CAD build for the part. Positions are in the model's coordinates, mm. A direction names the side the tool comes from. Give positions to 0.01 mm unless a question says otherwise; leave off trailing zeros. Loops run counter-clockwise (first coordinate to the right, second up) from the corner with the lowest first, then second, coordinate; pieces in that order, holes last.
```python
from build123d import *

# Parameters (mm, degrees)
SKETCH1_R           = 44.45
BOSS_EXTRUDE1_DEPTH = 6.35
BOSS_EXTRUDE4_DEPTH = 34.036
SKETCH3_R           = 2.6416
CUT_EXTRUDE1_DEPTH  = 75.717026145


with BuildPart() as part:
    # Sketch1 → Boss-Extrude1 (new body)
    with BuildSketch(Plane.XY):
        Circle(SKETCH1_R)
    extrude(amount=BOSS_EXTRUDE1_DEPTH)

    # Sketch2 → Boss-Extrude4 (add)
    with BuildSketch(Plane.XY.offset(6.35)):
        with BuildLine():
            Line((-2.1971, 17.145), (2.1971, 17.145))
            Line((2.1971, 17.145), (2.1971, 13.081))
            ThreePointArc((2.1971, 13.081), (0, -13.264230449), (-2.1971, 13.081))
            Line((-2.1971, 13.081), (-2.1971, 17.145))
        make_face()
    extrude(amount=BOSS_EXTRUDE4_DEPTH)

    # Sketch3 → Cut-Extrude1 (cut, through all)
    with BuildSketch(Plane(origin=(0, 0, 0), x_dir=(-1, 0, 0), z_dir=(0, 0, -1))):
        Circle(SKETCH3_R)
    extrude(amount=-CUT_EXTRUDE1_DEPTH, mode=Mode.SUBTRACT)


solid = part.part
```
1. Saw through at C-C, the plane y = 0. List the corners of the cut face in (x, z).
Responses:
outline: (-44.45, 0) - (-2.64, 0) - (-2.64, 40.39) - (-13.26, 40.39) - (-13.26, 6.35) - (-44.45, 6.35) - close; (2.64, 0) - (44.45, 0) - (44.45, 6.35) - (13.26, 6.35) - (13.26, 40.39) - (2.64, 40.39) - close
2. Drop flat-ended pins along their axis: pin 1 (5 mm diameter, centred on x = 11, z = 11.5, fed in from -Y); pin 2 (8.5 mm diameter, centred on x = 0, y = 0, fed in from +Z); pin 3 (5 mm diameter, centred on x = 1, z = 26.5, fed in from +Y) (3 decimals); pin 4 (12 mm diameter, centred on x = 2.5, y = 32.5, fed in from +Z). Give the stop position or say it passes through.
Responses:
pin 1: stops at y = -10.18
pin 2: stops at z = 40.39
pin 3: stops at y = 17.145
pin 4: stops at z = 6.35
3. Pull direction Y, two halves, no side cores. Call faces 5 (the face through (0.552, -13.253, 23.13)), 6 (the face through (2.1, -1.6, 19.9)), 7 (the face through (-1, -9, 0)): released by +Y, released by -Y, zero draft, split by the parting line, or undercut.
Responses:
face 5: split by the parting line
face 6: undercut
face 7: zero draft
4. Probe line 1 along Y through (x, z) = (0, 21) (3 decimals); line 2 along Z through (x, y) = (16.5, 17); line 3 along X through (y, z) = (9, 8.5). List the from-to ranges inside material, lowest first.
Responses:
line 1: y = -13.264 to -2.642, 2.642 to 17.145
line 2: z = 0 to 6.35
line 3: x = -9.74 to 9.74
5. Saw through at A-A, the plane x = 0. List the corners of the cut face in (y, z) (3 decimals).
Responses:
outline: (-44.45, 0) - (-2.642, 0) - (-2.642, 40.386) - (-13.264, 40.386) - (-13.264, 6.35) - (-44.45, 6.35) - close; (2.642, 0) - (44.45, 0) - (44.45, 6.35) - (17.145, 6.35) - (17.145, 40.386) - (2.642, 40.386) - close
6. Saw through at B-B, the plane z = 17. List the corners of the cut face in (x, y) (3 decimals), and give its area (3 significant figures).
Responses:
outline: (-2.197, 13.081) arc R13.264 ccw (long way) to (2.197, 13.081) - (2.197, 17.145) - (-2.197, 17.145) - close; hole circle Ø5.283 at (0, 0)
area: 548 mm2
7. Tool access for faces 1 (the face through (42.397, 13.352, 3.131)), 2 (the face through (-2.197, 15, 23)), 3 (the face through (2.197, 15, 23)), 4 (the face through (0, 17.145, 23)): list every direction of +Z, -Z, +X, -X, +Y, -Y with a clear straight run to the whole face (end or side of a thin tool).
Responses:
face 1: +Z, -Z
face 2: +Z, -X, +Y
face 3: +Z, +X, +Y
face 4: +Z, +X, -X, +Y
8. Saw through at D-D, the plane x = -11. List the corners of the cut face in (y, z).
Responses:
outline: (-43.07, 0) - (43.07, 0) - (43.07, 6.35) - (7.41, 6.35) - (7.41, 40.39) - (-7.41, 40.39) - (-7.41, 6.35) - (-43.07, 6.35) - close
